Verification items for the finished model (mm, model axes). A direction names the side the tool comes from. Give positions to 0.01 mm unless a question says otherwise; leave off trailing zeros. Write each loop counter-clockwise with the first axis right and the second up, starting at its lowest first coordinate (ties: lowest second). Pieces come first, ordered by that corner, then holes. Notation, with made-up numbers: (29.25, -20) -> (56.25, -20) arc R17 cw to (56.25, -15) -> close; hole circle Ø9 at (-11.75, 8). An arc over 180 degrees is marked (long way). Answer as CSV lines item,"result".
```python
from build123d import *

# Parameters (mm, degrees)
ESQUISSE1_W             = 33
ESQUISSE1_H             = 2
BOSS_EXTRU_1_REACH      = 80.689
ESQUISSE5_R             = 16.5
ESQUISSE5_R_2           = 13.5
ENL_V_MAT_EXTRU_1_REACH = 80.689
ESQUISSE6_R             = 13.5


with BuildPart() as part:
    # Esquisse1 → Révolution1 (revolve)
    with BuildSketch(Plane.XY, mode=Mode.PRIVATE) as r_volution1_sk:
        with Locations((0, -1)):
            Rectangle(ESQUISSE1_W, ESQUISSE1_H)
    revolve(r_volution1_sk.sketch.rotate(Axis((0, -23, 0), (1, 0, 0)), 90), axis=Axis((0, -23, 0), (1, 0, 0)))

    # Esquisse5 → Boss.-Extru.1 (add, up to next)
    with BuildSketch(Plane.XZ, mode=Mode.PRIVATE) as boss_extru_1_sk1:
        with Locations(Location((0, 0, 0), (0, 0, 180))):
            Circle(ESQUISSE5_R)
        with Locations(Location((0, 0, 0), (0, 0, 180))):
            Circle(ESQUISSE5_R_2, mode=Mode.SUBTRACT)
    boss_extru_1_tool1 = extrude(boss_extru_1_sk1.sketch, amount=BOSS_EXTRU_1_REACH, mode=Mode.PRIVATE) - part.part


with BuildPart() as body_2:
    # Esquisse2 → Révolution2 (revolve)
    with BuildSketch(Plane.XY):
        Polygon((-16.5, 0), (-16.5, 25), (-36, 25), (-36, 27.5), (-16.5, 27.5), (-16.5, 31.5), (-36, 31.5), (-36, 34), (-16.5, 34), (-16.5, 38), (-36, 38), (-36, 40.5), (-23.5, 40.5), (-23.5, 44.5), (-36, 44.5), (-36, 47), (-23.5, 47), (-23.5, 51), (-36, 51), (-36, 53.5), (-23.5, 53.5), (-23.5, 57.5), (-36, 57.5), (-36, 60), (0, 60), (0, 56), (-13.5, 56), (-13.5, 0), align=None)
    revolve(axis=Axis((0, 56, 0), (0, -1, 0)))

    # Esquisse4 → Enlèvement de matière-Révolution1 (revolve, cut)
    with BuildSketch(Plane.XY, mode=Mode.PRIVATE) as enl_vement_de_mati_re_r_volution1_sk:
        Polygon((-36, 60), (-36, 53.5), (-30.5, 25), (-37, 25), (-37, 60), align=None)
    revolve(enl_vement_de_mati_re_r_volution1_sk.sketch.rotate(Axis((0, 0, 0), (0, 1, 0)), 180), axis=Axis((0, 0, 0), (0, 1, 0)), mode=Mode.SUBTRACT)


with BuildPart() as part_1:
    add(part.part)

    add(body_2.part)  # Boss.-Extru.1 merges body 2
    add(boss_extru_1_tool1.solids().sort_by_distance((16.03331, 0, 0))[0])
    add(boss_extru_1_tool1.solids().sort_by_distance((16.03331, 0, 0))[1])

    # Esquisse6 → Enlèv. mat.-Extru.1 (cut, up to next)
    with BuildSketch(Plane(origin=(0, 0, 0), x_dir=(1, 0, 0), z_dir=(0, 1, 0)), mode=Mode.PRIVATE) as enl_v_mat_extru_1_sk1:
        with Locations(Location((0, 0, 0), (0, 0, 180))):
            Circle(ESQUISSE6_R)
    enl_v_mat_extru_1_tool1 = extrude(enl_v_mat_extru_1_sk1.sketch, amount=-ENL_V_MAT_EXTRU_1_REACH, mode=Mode.PRIVATE) & part_1.part
    add(enl_v_mat_extru_1_tool1.solids().sort_by_distance((0, 0, 0))[0], mode=Mode.SUBTRACT)


solid = part_1.part
```
1) Depth check by flat-ended pin: pin 1 (2 mm diameter, centred on x = -5, z = -13, fed in from -Y); pin 2 (4 mm diameter, centred on y = 44.5, z = 21, fed in from -X); pin 3 (3 mm diameter, centred on x = -20.5, y = 24.5, fed in from -Z). Enter the tip coordinate at first touch or a pass-through.
Reported:
pin 1,"y = -42.62"
pin 2,"x = -28.59"
pin 3,"z = -23.79"
2) Tool access check on faces 4 (the cylindrical face through (4.686, 58.768, -35.694)), 5 (the flat face through (16.5, -13, -19)), 6 (the flat face through (-7, 53.5, 23)). Record the directions out of +Z, -Z, +X, -X, +Y, -Y that give a thin tool (end or side, any length) a straight path to the whole face; none if there is none.
Reported:
face 4,"+Y, -Y"
face 5,"+Z, -Z, +X, -Y"
face 6,"none"
3) Section check C-C (z = 19). State how many separate pieces and enclosed holes the cut face has, and give its area (3 significant figures).
Reported:
separate pieces,"5"
enclosed holes,"0"
area,"1,430 mm²"
4) Section check A-A (y = -23). Record the boundary of the cut face in (x, z).
Reported:
outline,"(-16.5, -23) -> (16.5, -23) -> (16.5, -21) -> (-16.5, -21) -> close; (-16.5, 21) -> (16.5, 21) -> (16.5, 23) -> (-16.5, 23) -> close"
5) Scan lines: line 1 along Y through (x, z) = (27.5, 11.5); line 2 along Y through (x, z) = (30, -15); line 3 along Y through (x, z) = (-20, 24). Record each from-to range of solid material in increasing order.
Reported:
line 1,"25 to 27.5, 31.5 to 34, 38 to 40.5, 44.5 to 47, 51 to 53.5, 57.5 to 60"
line 2,"44.5 to 47, 51 to 53.5, 57.5 to 60"
line 3,"31.5 to 34, 38 to 40.5, 44.5 to 47, 51 to 53.5, 57.5 to 60"
6) Draft check along Y on faces 1 (the cylindrical face through (-22.4, 42.5, -7.1)), 2 (the flat face through (-16.5, -13, -19)), 3 (the flat face through (1, 60, -1)). Enter one of: +Y half, -Y half, draft (parallel to the pull), parting line (faces both ways), or undercut.
Reported:
face 1,"undercut"
face 2,"draft"
face 3,"+Y half"
7) Section check B-B (y = 9.5). Record the boundary of the cut face in (x, z), and give its area (3 significant figures).
Reported:
outline,"circle Ø33 at (0, 0); hole circle Ø27 at (0, 0)"
area,"283 mm²"
